Autodesk Inventor part; units mm, degrees
ref_plane "YZ Plane" through (0, 0, 0) normal (1, 0, 0) x (0, 1, 0)
ref_plane "XZ Plane" through (0, 0, 0) normal (0, 1, 0) x (-1, 0, 0)
ref_plane "XY Plane" through (0, 0, 0) normal (0, 0, 1) x (1, 0, 0)
sketch "Skizze1" plane through (0, 0, 0) normal (1, 0, 0) x (0, 1, 0)
  arc A0 (250, 65.0592) -> (229.3412, 89.6794) centre (225, 65.0592) ccw
  line L0 (225, 65.0592) -> (229.3412, 89.6794) construction
  line L1 (225, 65.0592) -> (250, 65.0592) construction
  line L2 (229.3412, 89.6794) -> (0, 130.1185)
  line L3 (0, 130.1185) -> (0, 90.1185)
  arc A1 (229.3412, 40.439) -> (250, 65.0592) centre (225, 65.0592) ccw
  line L4 (229.3412, 40.439) -> (0, 0)
  line L5 (0, 0) -> (92.864, 0) construction
  line L6 (0, 0) -> (0, 40)
  line L7 (160, 76.5205) -> (160, 53.598)
  line L8 (40, 90.1185) -> (40, 40)
  line L9 (50, 40) -> (50, 90.1185)
  line L10 (82.882, 90.1185) -> (160, 76.5205)
  line L11 (82.882, 40) -> (160, 53.598)
  line L12 (0, 40) -> (40, 40)
  line L13 (50, 40) -> (82.882, 40)
  line L14 (0, 90.1185) -> (40, 90.1185)
  line L15 (50, 90.1185) -> (82.882, 90.1185)
  dimension "d21" = 80
  dimension "d24" = 25
  dimension "d68" = 250
  dimension "d73" = 80
  dimension "d88" = 130.1185
  dimension "d91" = 10
  dimension "d92" = 25
  dimension "d93" = 25
  dimension "d94" = 40
  dimension "d127" = 110
  dimension "d160" = 40
  dimension "d161" = 40
  dimension "d162" = 80
  dimension "d163" = 32.882
  dimension "d164" = 32.882
extrude "Extrusion2" add sketch "Skizze1" along normal blind 10
sketch "Skizze7" plane through (10, 0, 0) normal (1, 0, 0) x (0, 0, -1)
  arc A0 (-40.439, 229.3412) -> (-89.6794, 229.3412) centre (-65.0592, 225) ccw
  point P0 (0, 0)
hole "Bohrung6" at (10, 225, 65.0592) direction (-1, 0, 0) diameter 14 end through all
fillet "Rundung1" radius 2 5 edges at (5, 160, 76.5205) (5, 40, 90.1185) (5, 50, 40) (5, 160, 53.598) (5, 40, 40)
sketch "Skizze13" plane through (0, 0, 0) normal (-1, 0, 0) x (0, 0, 1)
  line L0 (80.5592, 240.5) -> (80.5592, 209.5)
  line L1 (80.5592, 209.5) -> (49.5592, 209.5)
  line L2 (49.5592, 209.5) -> (49.5592, 240.5)
  line L3 (49.5592, 240.5) -> (80.5592, 240.5)
  line L4 (80.5592, 240.5) -> (49.5592, 209.5) construction
  line L5 (80.5592, 209.5) -> (49.5592, 240.5) construction
  line L6 (80.5592, 240.5) -> (111.5592, 240.5) construction
  point P0 (0, 0)
  point P1 (65.0592, 225)
  dimension "d145" = 31
  dimension "d146" = 90
  dimension "d147" = 31
hole "Bohrung10" at (0, 209.5, 80.5592) at (0, 240.5, 80.5592) at (0, 240.5, 49.5592) at (0, 209.5, 49.5592) direction (1, 0, 0) diameter 3 end through all counterbore diameter 5 counterbore depth 5
sketch "Skizze14" plane through (10, 0, 0) normal (1, 0, 0) x (0, 0, -1)
  line L0 (-90.1185, 0) -> (-90.1185, 38)
  line L1 (-90.1185, 0) -> (-100.1185, 0)
  line L2 (-100.1185, 0) -> (-100.1185, 80)
  line L3 (-100.1185, 80) -> (-90.1185, 80)
  line L4 (-90.1185, 80) -> (-90.1185, 0)
  line L5 (-40, 0) -> (0, 0)
  line L6 (-40, 0) -> (-30, 0)
  line L7 (-30, 0) -> (-30, 80)
  line L8 (-30, 80) -> (-40, 80)
  line L9 (-40, 80) -> (-40, 0)
  dimension "d165" = 10
  dimension "d166" = 80
  dimension "d167" = 10
  dimension "d168" = 80
sketch "Skizze15" plane through (10, 0, 0) normal (1, 0, 0) x (0, 0, -1)
  circle A0 centre (-65.0592, 225) radius 7
  circle A1 centre (-65.0592, 225) radius 12
  point P0 (0, 0)
  dimension "d157" = 24
extrude "Extrusion4" cut sketch "Skizze15" against normal blind 5
sketch "Skizze16" plane through (10, 0, 0) normal (1, 0, 0) x (0, 0, -1)
  point P0 (0, 0)
sketch "Skizze17" plane through (10, 0, 0) normal (1, 0, 0) x (0, 0, -1)
  point P0 (0, 0)
extrude "Extrusion5" add sketch "Skizze14" along normal blind 20
sketch "Skizze18" plane through (10, 0, 100.1185) normal (0, 0, 1) x (1, 0, 0)
  line L0 (0, 0) -> (0, 80)
  line L1 (0, 0) -> (20, 0)
  line L2 (20, 80) -> (20, 0)
  line L3 (0, 80) -> (20, 80)
  line L4 (20, 80) -> (20, 0)
  line L5 (20, 0) -> (0, 80)
  line L6 (20, 80) -> (0, 80)
  point P0 (-10, 0)
sketch "Skizze19" plane through (10, 0, 0) normal (1, 0, 0) x (0, 0, -1)
  line L0 (0, 0) -> (-40.439, 229.3412)
  arc A0 (-40.439, 229.3412) -> (-89.6794, 229.3412) centre (-65.0592, 225) ccw
  line L1 (-89.6794, 229.3412) -> (-130.1185, 0)
  line L2 (-130.1185, 0) -> (-100.1185, 0)
  line L3 (-100.1185, 0) -> (-100.1185, 80)
  line L4 (-90.1185, 80) -> (-90.1185, 82.882)
  line L5 (-90.1185, 82.882) -> (-76.8119, 158.3473)
  arc A1 (-74.8423, 160) -> (-76.8119, 158.3473) centre (-74.8423, 158) ccw
  line L6 (-74.8423, 160) -> (-55.2762, 160)
  arc A2 (-53.3066, 158.3473) -> (-55.2762, 160) centre (-55.2762, 158) ccw
  line L7 (-53.3066, 158.3473) -> (-40, 82.882)
  line L8 (-40, 82.882) -> (-40, 80)
  line L9 (-30, 80) -> (-30, 0)
  line L10 (-30, 0) -> (0, 0)
  circle A3 centre (-65.0592, 225) radius 12
  circle A4 centre (-49.5592, 240.5) radius 1.5
  circle A5 centre (-80.5592, 209.5) radius 1.5
  circle A6 centre (-80.5592, 240.5) radius 1.5
  circle A7 centre (-49.5592, 209.5) radius 1.5
  line L11 (-90.1185, 80) -> (-90.1185, 0)
  line L12 (-105.1185, 80) -> (-90.1185, 80)
  line L13 (-105.1185, 0) -> (-105.1185, 80)
  line L14 (-105.1185, 0) -> (-90.1185, 0)
  line L15 (-130.1185, 0) -> (-105.1185, 0)
  line L16 (-100.1185, 0) -> (-100.1185, 80)
  line L17 (-100.1185, 0) -> (-100.1185, 5)
  line L18 (-100.1185, 0) -> (-95.1185, 0) construction
  line L19 (-100.1185, 5) -> (-129.2368, 5)
  line L20 (-130.1185, 0) -> (-129.2368, 5)
  line L21 (-100.1185, 80) -> (-90.1185, 80)
  line L22 (-40, 80) -> (-30, 80)
  dimension "d173" = 5
  dimension "d174" = 90
sketch "Skizze20" plane through (10, 0, 0) normal (1, 0, 0) x (0, 0, -1)
  point P0 (0, 0)
extrude "Extrusion7" add sketch "Skizze19" along normal blind 20 contours L19 L13 L2 L1 | L19 L3 L2 L13
sketch "Skizze21" plane through (10, 0, 0) normal (1, 0, 0) x (0, 0, -1)
  circle A0 centre (-49.5592, 209.5) radius 1.5
  circle A1 centre (-80.5592, 240.5) radius 1.5
  circle A2 centre (-80.5592, 209.5) radius 1.5
  circle A3 centre (-49.5592, 240.5) radius 1.5
  circle A4 centre (-65.0592, 225) radius 12
  line L0 (-129.2368, 5) -> (-100.1185, 5)
  line L1 (-100.1185, 5) -> (-100.1185, 80)
  line L2 (-100.1185, 80) -> (-90.1185, 80)
  line L3 (-90.1185, 80) -> (-90.1185, 82.882)
  line L4 (-90.1185, 82.882) -> (-76.8119, 158.3473)
  arc A5 (-74.8423, 160) -> (-76.8119, 158.3473) centre (-74.8423, 158) ccw
  line L5 (-74.8423, 160) -> (-55.2762, 160)
  arc A6 (-53.3066, 158.3473) -> (-55.2762, 160) centre (-55.2762, 158) ccw
  line L6 (-53.3066, 158.3473) -> (-40, 82.882)
  line L7 (-40, 82.882) -> (-40, 80)
  line L8 (-40, 80) -> (-30, 80)
  line L9 (-30, 80) -> (-30, 0)
  line L10 (-30, 0) -> (0, 0)
  line L11 (0, 0) -> (-40.439, 229.3412)
  arc A7 (-40.439, 229.3412) -> (-89.6794, 229.3412) centre (-65.0592, 225) ccw
  line L12 (-89.6794, 229.3412) -> (-129.2368, 5)
  line L13 (-40, 0) -> (-30, 0)
  line L14 (-30, 0) -> (-30, 80)
  line L15 (-30, 80) -> (-40, 80)
  line L16 (-40, 80) -> (-40, 0)
  line L17 (0, 0) -> (-0.8816, 5)
  line L18 (-30, 80) -> (-30, 0)
  line L19 (-30, 5) -> (-30, 0)
  line L20 (-30, 0) -> (0, 0)
  line L21 (-30, 5) -> (-0.8816, 5)
  dimension "d177" = 5
extrude "Extrusion8" add sketch "Skizze21" along normal blind 20 contours L11 L10 L9 L21
extrude "Extrusion9" cut sketch "Skizze18" along normal through all both and the other way through all contours L3 L2 L5
sketch "Skizze22" plane through (10, 5, 30) normal (0, 1, 0) x (1, 0, 0)
  line L0 (0, -60.1185) -> (20, -60.1185) construction
  line L1 (20, -100.1185) -> (20, -60.1185) construction
  line L2 (20, -10) -> (20, 30) construction
  line L3 (20, -10) -> (0, -10) construction
  point P0 (-10, 30)
  point P1 (10, -85.1185)
  point P2 (10, 15)
  dimension "d182" = 25
  dimension "d183" = 10
  dimension "d184" = 10
  dimension "d185" = 25
hole "Bohrung11" at (20, 5, 115.1185) at (20, 5, 15) direction (0, -1, 0) diameter 6.3 end through all
fillet "Rundung2" radius 2 5 edges at (10, 44, 90.1185) (5, 50, 90.1185) (29.375, 2.5, 0.4408) (29.375, 2.5, 129.6777) (10, 45, 40)
sketch "Skizze23" plane through (0, 0, 0) normal (-1, 0, 0) x (0, 0, 1)
  circle A0 centre (80.5592, 240.5) radius 2.5
  circle A1 centre (80.5592, 240.5) radius 5
  circle A2 centre (49.5592, 240.5) radius 2.5
  circle A3 centre (49.5592, 240.5) radius 5
  arc A4 (89.6794, 229.3412) -> (40.439, 229.3412) centre (65.0592, 225) ccw
  point P0 (0, 0)
  dimension "d194" = 10
  dimension "d195" = 10
extrude "Extrusion10" add sketch "Skizze23" against normal blind 10
ref_plane "Arbeitsebene4" through (0, 245, 90.1185) normal (0, -1, 0) x (1, 0, 0)
sketch "Skizze24" plane through (0, 245, 90.1185) normal (0, -1, 0) x (1, 0, 0)
  line L0 (-28.75, 54.9898) -> (28.75, 54.9898)
  line L1 (28.75, 54.9898) -> (28.75, -54.9898)
  line L2 (28.75, -54.9898) -> (-28.75, -54.9898)
  line L3 (-28.75, -54.9898) -> (-28.75, 54.9898)
  line L4 (12, 0) -> (0, 0)
  line L5 (-28.75, 54.9898) -> (28.75, -54.9898) construction
  line L6 (28.75, 54.9898) -> (-28.75, -54.9898) construction
  point P0 (0, -90.1185)
  dimension "d199" = 57.5
  dimension "d200" = 109.9796
extrude "Extrusion11" cut sketch "Skizze24" against normal blind 10
properties part number "halter_seite_motor"
Design review of the part built by this model. Coordinates are the model's own, in mm. A direction names the side the tool comes from. Give positions to 0.01 mm unless a question says otherwise; leave off trailing zeros. Loops run counter-clockwise (first coordinate to the right, second up) from the corner with the lowest first, then second, coordinate; pieces in that order, holes last. Notation, with made-up numbers: M -40,83 L 9,83 A20 cw 9,108 Z; hole C -26.75,9.5 d9. An arc over 180 degrees is marked long. Return JSON: item names as keys, results as strings. Group by question number.
Item 1: We need section D-D (y = 225). Give the boundary of the cut face in (x, z), and give its area (3 significant figures).
Item 2: We need section A-A (x = 20). Give the boundary of the cut face in (y, z).
Item 3: Tool access review of faces 4 (the flat face through (5, 160, 65)), 5 (the flat face through (17, 34, 100.118)), 6 (the cylindrical face through (2.54, 238.02, 80.23)), 7 (the cylindrical face through (7.5, 236.9, 66.6)), 8 (the flat face through (10, 123, 37)): name each direction out of +Z, -Z, +X, -X, +Y, -Y from which nothing blocks a thin tool from reaching the whole face with its end or side.
Item 4: For probe 1 along Z at (x, y) = (6.5, 240.5); probe 2 along Z at (x, y) = (7.4, 209.5); probe 3 along X at (y, z) = (164, 55), list the stretches that pass through material, from the lowest coordinate up.
Item 5: Insertion check: pin 1 Ø9.5 at (x, z) = (17, 112.5) entering from +Y; pin 2 Ø11 at (x, z) = (7, 68) entering from -Y; pin 3 Ø9 at (x, y) = (8.5, 51) entering from +Z; pin 4 Ø2.5 at (y, z) = (240.5, 49.56) entering from -X (1 decimal). Each pin has a flat end and moves straight along its axis. Give the tip position at first contact, or say it passes through.
Item 6: We need section C-C (y = 73). Give the boundary of the cut face in (x, z), and give its area (3 significant figures).
Item 7: We need section B-B (z = 15). Give the boundary of the cut face in (x, y), and give its area (3 significant figures).
Item 8: Mouldability with a two-part tool opening along Z and no side actions: class faces 1 (the flat face through (5.643, 106.712, 111.302)), 2 (the flat face through (10, 45, 65)), 3 (the flat face through (19, 5, 19)) as released by +Z, released by -Z, zero draft, split by the parting line, or undercut.
Output:
{
 "1": {"outline": "M 0,39.67 L 10,39.67 L 10,53.06 L 5,53.06 L 5,58.06 L 0,58.06 Z; M 0,72.06 L 5,72.06 L 5,77.06 L 10,77.06 L 10,90.44 L 0,90.44 Z", "area": "318 mm^2"},
 "2": {"outline": "M 0,0 L 5,0.88 L 5,11.85 L 0,11.85 Z; M 0,18.15 L 5,18.15 L 5,30 L 40,30 L 40,40 L 0,40 Z; M 0,90.12 L 40,90.12 L 40,100.12 L 5,100.12 L 5,111.97 L 0,111.97 Z; M 0,118.27 L 5,118.27 L 5,129.24 L 0,130.12 Z"},
 "3": {"face 4": "+X, -X", "face 5": "+Z, +X, +Y", "face 6": "-X", "face 7": "+X", "face 8": "+X, +Y"},
 "4": {"probe 1": "z = 44.56 to 48.06, 51.06 to 79.06, 82.06 to 85.56", "probe 2": "z = 36.94 to 48.06, 51.06 to 79.06, 82.06 to 93.18", "probe 3": "x = 0 to 10"},
 "5": {"pin 1": "stops at y = 5", "pin 2": "stops at y = 40", "pin 3": "stops at z = 121.92", "pin 4": "passes through"},
 "6": {"outline": "M 0,12.87 L 10,12.87 L 10,30 L 11.75,30 L 11.75,40 L 0,40 Z; M 0,90.12 L 11.75,90.12 L 11.75,100.12 L 10,100.12 L 10,117.25 L 0,117.25 Z", "area": "578 mm^2"},
 "7": {"outline": "M 0,0 L 16.85,0 L 16.85,5 L 10,5 L 10,85.07 L 0,85.07 Z; M 23.15,0 L 30,0 L 28.75,5 L 23.15,5 Z", "area": "916 mm^2"},
 "8": {"face 1": "released by +Z", "face 2": "undercut", "face 3": "zero draft"}
}
